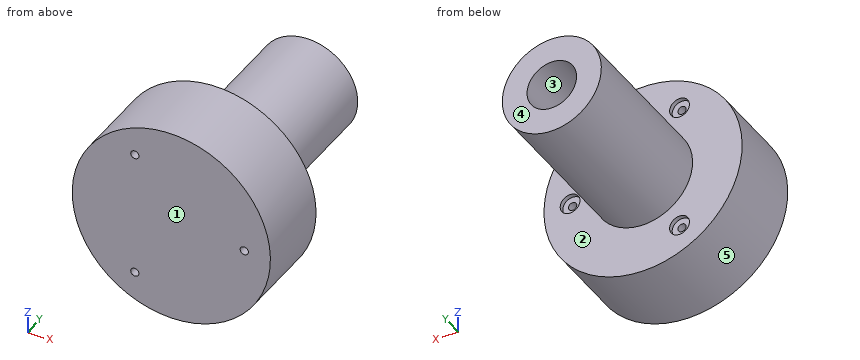
from build123d import *

# Parameters (mm, degrees)
SKETCH1_R                                           = 7.9375
BOSS_EXTRUDE1_DEPTH                                 = 25.4
SKETCH2_R                                           = 15.875
BOSS_EXTRUDE2_DEPTH                                 = 12.7
SKETCH3_R                                           = 3.96875
CUT_EXTRUDE1_DEPTH                                  = 19.05
CBORE_FOR_00_BINDING_HEAD_MACHINE_SCREW_D           = 1.3208
CBORE_FOR_00_BINDING_HEAD_MACHINE_SCREW_CBORE_D     = 3.175
CBORE_FOR_00_BINDING_HEAD_MACHINE_SCREW_CBORE_DEPTH = 0.7112
CIRPATTERN1_COUNT                                   = 3


with BuildPart() as part:
    # Sketch1 → Boss-Extrude1 (new body)
    with BuildSketch(Plane(origin=(0, 0, 0), x_dir=(1, 0, 0), z_dir=(0, 1, 0))):
        with Locations(Location((0, 0, 0), (0, 0, 270))):
            Circle(SKETCH1_R)
    extrude(amount=BOSS_EXTRUDE1_DEPTH)

    # Sketch2 → Boss-Extrude2 (add)
    with BuildSketch(Plane(origin=(0, 0, 0), x_dir=(-1, 0, 0), z_dir=(0, -1, 0))):
        with Locations(Location((0, 0, 0), (0, 0, 90))):
            Circle(SKETCH2_R)
    extrude(amount=BOSS_EXTRUDE2_DEPTH)

    # Sketch3 → Cut-Extrude1 (cut)
    with BuildSketch(Plane(origin=(0, 25.4, 0), x_dir=(1, 0, 0), z_dir=(0, 1, 0))):
        with Locations(Location((0, 0, 0), (0, 0, 270))):
            Circle(SKETCH3_R)
    extrude(amount=-CUT_EXTRUDE1_DEPTH, mode=Mode.SUBTRACT)

    # CBORE for #00 Binding Head Machine Screw1 (through all)
    with Locations(Plane(origin=(0, 0, 0), x_dir=(1, 0, 0), z_dir=(0, 1, 0))):
        with Locations((11.687693986, 0)):
            cbore_for_00_binding_head_machine_screw = CounterBoreHole(CBORE_FOR_00_BINDING_HEAD_MACHINE_SCREW_D / 2, CBORE_FOR_00_BINDING_HEAD_MACHINE_SCREW_CBORE_D / 2, CBORE_FOR_00_BINDING_HEAD_MACHINE_SCREW_CBORE_DEPTH)

    # CirPattern1: CBORE for #00 Binding Head Machine Screw1 ×3 about axis
    cirpattern1_axis = Axis((0, 0, 0), (0, 1, 0))
    for i in range(1, CIRPATTERN1_COUNT):
        add(cbore_for_00_binding_head_machine_screw.rotate(cirpattern1_axis, i * 360 / CIRPATTERN1_COUNT), mode=Mode.SUBTRACT)


solid = part.part
Verification items for the finished model (mm, model axes). Face numbers are marked on the shaded views. A direction names the side the tool comes from. Give positions to 0.01 mm unless a question says otherwise; leave off trailing zeros. Write each loop counter-clockwise with the first axis right and the second up, starting at its lowest first coordinate (ties: lowest second). Pieces come first, ordered by that corner, then holes. Notation, with made-up numbers: M 75,37 L 88,37 A20 ccw 88,56 Z; hole C 29.5,87.5 d2. An arc over 180 degrees is marked long. Put each result on its own line as item: value. Start each with the question number.
1. Section check C-C (y = 8). Record the cut outline in (x, z) (1 decimal), and give its area (3 significant figures).
2. Set-up check for the marked faces 1 and 2: record each of +Z, -Z, +X, -X, +Y, -Y from which the full face is reachable in a straight line by a thin tool's end or side.
3. Scan lines: line 1 along Y through (x, z) = (-12, -7); line 2 along Y through (x, z) = (12, -1.5); line 3 along X through (y, z) = (15, 3). Record each from-to range of solid material in increasing order. Write a range as [from, to].
4. Section check D-D (z = 13.5). Record the cut outline in (x, y).
5. Draft check along Z on the marked faces 3, 4 and 5. Enter one of: +Z half, -Z half, draft (parallel to the pull), parting line (faces both ways), or undercut.
6. Go/stop test with flat-tipped pins: pin 1 Ø2.5 at (x, z) = (-6.5, 10) entering from +Y; pin 2 Ø2 at (y, z) = (14.5, 1) entering from +X; pin 3 Ø1.1 at (x, z) = (-5.84, -10.12) entering from +Y; pin 4 Ø5 at (y, z) = (-0.5, -8) entering from +X. Record where each tip stops, or that it passes through.
Answer list:
1. outline: C 0,0 d15.9; hole C 0,0 d7.9
1. area: 148 mm2
2. face 1: +Z, -Z, +X, -X, -Y
2. face 2: +Y
3. line 1: [-12.7, 0]
3. line 2: [-12.7, -0.71]
3. line 3: [-7.35, -2.6], [2.6, 7.35]
4. outline: M -8.35,-12.7 L 8.35,-12.7 L 8.35,0 L -8.35,0 Z
5. face 3: undercut
5. face 4: draft
5. face 5: parting line
6. pin 1: y = 0
6. pin 2: x = 7.94
6. pin 3: through
6. pin 4: x = 14.89
